Could you check a few things on this drawing? It's one solid part, dimensions in mm from its lowest x, y, z. A direction names the side the tool comes from. Give positions to 0.01 mm unless a question says otherwise; leave off trailing zeros. Loops run counter-clockwise (first coordinate to the right, second up) from the corner with the lowest first, then second, coordinate; pieces in that order, holes last. Notation, with made-up numbers: (25, 60.25) - (59, 60.25) arc R30 cw to (59, 93.25) - close; hole circle Ø7 at (23.25, -33.75). An arc over 180 degrees is marked (long way). Write item = value, one per line.
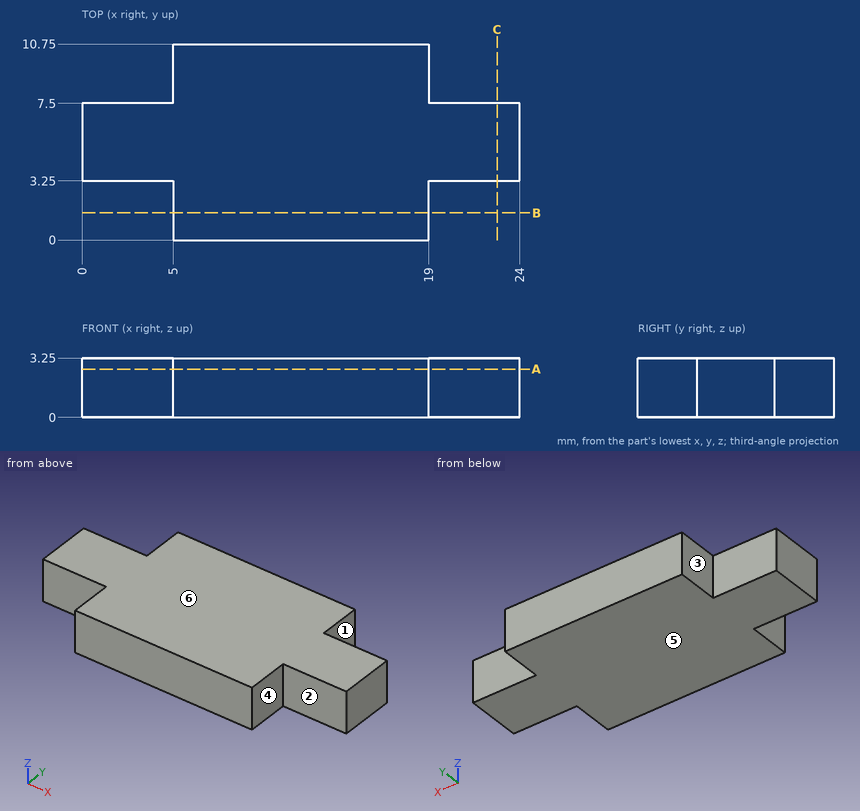
Q1. Imagine slicing it at C-C, the plane x = 22.75. Write out the boundary of the cut face in (y, z).
Output:
outline = (3.25, 0) - (7.5, 0) - (7.5, 3.25) - (3.25, 3.25) - close
Q2. I need wall thicknesses on L1, parallel to Y at x = 19.5, z = 0.2; L2, parallel to X at y = 0.5, z = 2.45. Which ranges of each line are inside material? Lowest first, please.
Output:
L1 = 3.25 to 7.5
L2 = 5 to 19
Q3. For pin 1 (1 mm diameter, centred on x = 2.5, z = 1, fed in from -Y); pin 2 (1 mm diameter, centred on y = 1.5, z = 1.5, fed in from +X); pin 3 (1 mm diameter, centred on y = 2.5, z = 1, fed in from -X), each with a flat end and sliding along its axis, tell me the tip position at first contact or that it passes through.
Output:
pin_1 = 3.25
pin_2 = 19
pin_3 = 5
Q4. Imagine slicing it at B-B, the plane y = 1.5. Write out the boundary of the cut face in (x, z), then the cut area to 3 significant figures.
Output:
outline = (5, 0) - (19, 0) - (19, 3.25) - (5, 3.25) - close
area = 45.5 mm2
Q5. We'd pull the mould along Z, two halves only. Please class the marked faces 4, 5 and 6: released by +Z, released by -Z, zero draft, split by the parting line, or undercut.
Output:
face_4 = zero draft
face_5 = released by -Z
face_6 = released by +Z
Q6. Which directions (+Z, -Z, +X, -X, +Y, -Y) give clear straight access to the entire face, cutting with the end or side of a thin tool? Please do the marked faces 1, 2 and 3.
Output:
face_1 = +Z, -Z, +X, +Y
face_2 = +Z, -Z, +X, -Y
face_3 = +Z, -Z, -X, +Y
Q7. Imagine slicing it at A-A, the plane z = 2.65. Write out the boundary of the cut face in (x, y).
Output:
outline = (0, 3.25) - (5, 3.25) - (5, 0) - (19, 0) - (19, 3.25) - (24, 3.25) - (24, 7.5) - (19, 7.5) - (19, 10.75) - (5, 10.75) - (5, 7.5) - (0, 7.5) - close
